from build123d import *

# Parameters (mm, degrees)
BOSS_EXTRUDE1_DEPTH     = 3
SKETCH2_R               = 1
CUT_EXTRUDE1_DEPTH      = 1
CUT_EXTRUDE1_DEPTH_BACK = 4


with BuildPart() as part:
    # Sketch1 → Boss-Extrude1 (new body)
    with BuildSketch(Plane.XY):
        with BuildLine():
            Line((-6, -30), (-14.580127019, -30))
            ThreePointArc((-14.580127019, -30), (-15.110457105, -29.780330086), (-15.330127019, -29.25))
            Line((-15.330127019, -29.25), (-15.330127019, -29.075495241))
            ThreePointArc((-15.330127019, -29.075495241), (-15.175142024, -28.618924169), (-14.774241303, -28.351050871))
            Line((-14.774241303, -28.351050871), (-11.188266684, -27.390191868))
            ThreePointArc((-11.188266684, -27.390191868), (-7.446526618, -24.890041087), (-6, -20.628711084))
            Line((-6, -20.628711084), (-6, 0))
            Line((-6, 0), (-6, 3))
            ThreePointArc((-6, 3), (-5.414213562, 4.414213562), (-4, 5))
            Line((-4, 5), (4, 5))
            ThreePointArc((4, 5), (5.414213562, 4.414213562), (6, 3))
            Line((6, 3), (6, 0))
            Line((6, 0), (6, -30))
            Line((6, -30), (-6, -30))
        make_face()
    extrude(amount=BOSS_EXTRUDE1_DEPTH)

    # Sketch2 → Cut-Extrude1 (cut, two sides)
    with BuildSketch(Plane.XY.offset(3)) as cut_extrude1_sk:
        Circle(SKETCH2_R)
    extrude(amount=CUT_EXTRUDE1_DEPTH, mode=Mode.SUBTRACT)
    extrude(cut_extrude1_sk.sketch, amount=-CUT_EXTRUDE1_DEPTH_BACK, mode=Mode.SUBTRACT)


solid = part.part
Geometry check sheet. Reference: the model listing, model coordinates, mm. A direction names the side the tool comes from. Round coordinates to 2 decimals unless told otherwise and drop trailing zeros. Order: outer loops, then holes, each group sorted by start corner. A loop starts at its lowest first (then second) coordinate and runs counter-clockwise, first axis right, second up. Notation, with made-up numbers: M 16.25,-20.75 L 37.25,-20.75 A24 ccw 37.25,2.25 Z; hole C -23.5,31 d10. An arc over 180 degrees is marked long. Answer in a Markdown table with one row per item.
(1) Sectioned sample at A-A, the plane z = 0.4. Record the cut outline in (x, y), and give its area (3 significant figures).
Responses:
| item | result |
|---|---|
| outline | M -15.33,-29.25 A0.75 ccw -14.58,-30 L 6,-30 L 6,3 A2 ccw 4,5 L -4,5 A2 ccw -6,3 L -6,-20.63 A7 cw -11.19,-27.39 L -14.77,-28.35 A0.75 ccw -15.33,-29.08 Z; hole C 0,0 d2 |
| area | 446 mm² |
(2) Scan lines: probe 1 along Y at (x, z) = (0, 1.05); probe 2 along X at (y, z) = (-2, 1.6); probe 3 along Y at (x, z) = (0.75, 2.45). Record each from-to range of solid material in increasing order. Write a range as from..to.
Responses:
| item | result |
|---|---|
| probe 1 | y = -30..-1, 1..5 |
| probe 2 | x = -6..6 |
| probe 3 | y = -30..-0.66, 0.66..5 |
(3) Sectioned sample at B-B, the plane x = 0. Record the cut outline in (y, z), and give its area (3 significant figures).
Responses:
| item | result |
|---|---|
| outline | M -30,0 L -1,0 L -1,3 L -30,3 Z; M 1,0 L 5,0 L 5,3 L 1,3 Z |
| area | 99.0 mm² |
(4) Sectioned sample at D-D, the plane y = -7.5. Record the cut outline in (x, z).
Responses:
| item | result |
|---|---|
| outline | M -6,0 L 6,0 L 6,3 L -6,3 Z |
(5) Go/stop test with flat-tipped pins: P1, Ø4, axis at x = 2, y = -11, coming from the -Z side; P2, Ø1, axis at y = -12, z = 0.5, coming from the -X side. Record where each tip stops, or that it passes through.
Responses:
| item | result |
|---|---|
| P1 | stops at z = 0 |
| P2 | stops at x = -6 |
(6) Sectioned sample at C-C, the plane y = 0. Record the cut outline in (x, z).
Responses:
| item | result |
|---|---|
| outline | M -6,0 L -1,0 L -1,3 L -6,3 Z; M 1,0 L 6,0 L 6,3 L 1,3 Z |
(7) Draft check along X on faces 3 (the face through (5.4, 4.43, 1.48)), 4 (the face through (-5.43, 4.4, 1.48)), 5 (the face through (0, -1, 2)). Enter one of: released by +X, released by -X, zero draft, split by the parting line, or undercut.
Responses:
| item | result |
|---|---|
| face 3 | released by +X |
| face 4 | released by -X |
| face 5 | undercut |
(8) Tool access check on faces 1 (the face through (6, -13, 1)), 2 (the face through (-6, -9, 1)). Record the directions out of +Z, -Z, +X, -X, +Y, -Y that give a thin tool (end or side, any length) a straight path to the whole face; none if there is none.
Responses:
| item | result |
|---|---|
| face 1 | +Z, -Z, +X, +Y, -Y |
| face 2 | +Z, -Z, -X, +Y |
